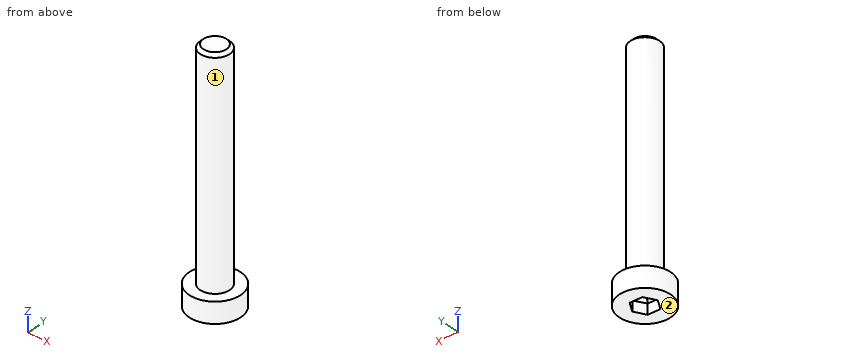
```python
from build123d import *

# Parameters (mm, degrees)
SKETCH_R        = 3.5
PAD_DEPTH       = 2.8
SKETCH001_R     = 2
PAD001_DEPTH    = 30
CHAMFER_SIZE    = 0.43
POCKET_DEPTH    = 2
CHAMFER001_SIZE = 0.6
SKETCH003_R     = 1.05
POCKET001_DEPTH = 1.5


with BuildPart() as part:
    # Sketch → Pad (new body)
    with BuildSketch(Plane.XY):
        Circle(SKETCH_R)
    extrude(amount=PAD_DEPTH)

    # Sketch001 → Pad001 (new body)
    with BuildSketch(Plane.XY.offset(2.8)):
        Circle(SKETCH001_R)
    extrude(amount=PAD001_DEPTH)

    # Chamfer
    chamfer_edges = [part.edges().sort_by_distance(p)[0] for p in [
        (-2, 0, 32.8),
    ]]
    chamfer(chamfer_edges, length=CHAMFER_SIZE)

    # Sketch002 → Pocket (cut)
    with BuildSketch(Plane(origin=(0, 0, 0), x_dir=(1, 0, 0), z_dir=(0, 0, -1))):
        Polygon((-0.866025, 1.5), (0.866025, 1.5), (1.732051, 0), (0.866025, -1.5), (-0.866025, -1.5), (-1.732051, 0), align=None)
    extrude(amount=-POCKET_DEPTH, mode=Mode.SUBTRACT)

    # Chamfer001
    chamfer001_edges = [part.edges().sort_by_distance(p)[0] for p in [
        (0, -1.5, 2),
        (1.299038, -0.75, 2),
        (1.299038, 0.75, 2),
        (0, 1.5, 2),
        (-1.299038, 0.75, 2),
        (-1.299038, -0.75, 2),
    ]]
    chamfer(chamfer001_edges, length=CHAMFER001_SIZE)

    # Sketch003 → Pocket001 (cut, symmetric)
    with BuildSketch(Plane(origin=(0, 0, 2), x_dir=(1, 0, 0), z_dir=(0, 0, -1))):
        Circle(SKETCH003_R)
    extrude(amount=POCKET001_DEPTH, both=True, mode=Mode.SUBTRACT)


solid = part.part
```
Verification items for the finished model (mm, model axes). Face numbers are marked on the shaded views. A direction names the side the tool comes from. Round coordinates to 2 decimals unless told otherwise and drop trailing zeros. Write each loop counter-clockwise with the first axis right and the second up, starting at its lowest first coordinate (ties: lowest second). Pieces come first, ordered by that corner, then holes. Notation, with made-up numbers: (8.25, 11.5) -> (38.25, 11.5) arc R8 ccw to (38.25, 21.5) -> close; hole circle Ø5 at (-27, 2.25). An arc over 180 degrees is marked (long way). Write each question's results on one line, items separated by ' | '. Start each with the question number.
1. Cross-section at C-C (y = -2.5). Enter the section's corners in (x, z), then the cut area to 3 significant figures.
2. Set-up check for the marked faces 1 and 2: record each of +Z, -Z, +X, -X, +Y, -Y from which the full face is reachable in a straight line by a thin tool's end or side.
3. Cross-section at D-D (x = 2.75). Enter the section's corners in (y, z).
4. Material ranges on probe 1 along Y at (x, z) = (0, 2.95); probe 2 along Y at (x, z) = (0, 2.7); probe 3 along Z at (x, y) = (-2.75, 1.75), recorded low to high. Write a range as from..to.
5. Cross-section at A-A (x = 0). Enter the section's corners in (y, z).
6. Cross-section at B-B (z = 27). Enter the section's corners in (x, y), then the cut area to 3 significant figures.
7. Depth check by flat-ended pin: P1, Ø1, axis at x = 0.5, z = 26.5, coming from the +Y side; P2, Ø1, axis at x = 2.5, y = -0.5, coming from the +Z side; P3, Ø1.5, axis at y = 1, z = 5, coming from the -X side; P4, Ø4, axis at x = 0, y = -2.5, coming from the +Z side. Enter the tip coordinate at first touch or a pass-through.
Solutions:
1) outline: (-2.45, 0) -> (2.45, 0) -> (2.45, 2.8) -> (-2.45, 2.8) -> close | area: 13.7 mm2
2) face 1: +Z | face 2: -Z, +X, -X, +Y, -Y
3) outline: (-2.17, 0) -> (2.17, 0) -> (2.17, 2.8) -> (-2.17, 2.8) -> close
4) probe 1: y = -2..-1.05, 1.05..2 | probe 2: y = -3.5..-1.05, 1.05..3.5 | probe 3: z = 0..2.8
5) outline: (-3.5, 0) -> (-1.5, 0) -> (-1.5, 1.4) -> (-1.05, 1.85) -> (-1.05, 3.5) -> (1.05, 3.5) -> (1.05, 1.85) -> (1.5, 1.4) -> (1.5, 0) -> (3.5, 0) -> (3.5, 2.8) -> (2, 2.8) -> (2, 32.37) -> (1.57, 32.8) -> (-1.57, 32.8) -> (-2, 32.37) -> (-2, 2.8) -> (-3.5, 2.8) -> close
6) outline: circle Ø4 at (0, 0) | area: 12.6 mm2
7) P1: stops at y = 2 | P2: stops at z = 2.8 | P3: stops at x = -1.98 | P4: stops at z = 32.8
